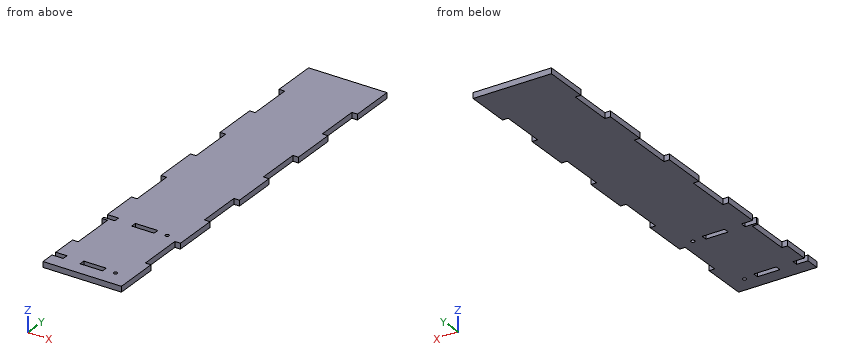
```python
from build123d import *

# Parameters (mm, degrees)
SKETCH2_W           = 6.35
SKETCH2_H           = 88.9
BOSS_EXTRUDE1_DEPTH = 457.2
SKETCH4_W           = 6.35
SKETCH4_H           = 50.8
CUT_EXTRUDE1_DEPTH  = 460.399570091
SKETCH5_W           = 12.7
SKETCH5_H           = 6.35
CUT_EXTRUDE2_DEPTH  = 460.399570091
SKETCH6_R           = 2.0955
CUT_EXTRUDE3_DEPTH  = 460.399570091
SKETCH7_W           = 12.7
SKETCH7_H           = 6.35
CUT_EXTRUDE4_DEPTH  = 10
SKETCH8_W           = 12.7
SKETCH8_H           = 6.35
CUT_EXTRUDE5_DEPTH  = 460.399570091


with BuildPart() as part:
    # Sketch2 → Boss-Extrude1 (new body)
    with BuildSketch(Plane.ZX):
        with Locations((41.275, 0)):
            Rectangle(SKETCH2_W, SKETCH2_H)
    extrude(amount=BOSS_EXTRUDE1_DEPTH)

    # Sketch4 → Cut-Extrude1 (cut, through all)
    with BuildSketch(Plane.XY.offset(44.45)):
        with Locations((41.275, 381)):
            Rectangle(SKETCH4_W, SKETCH4_H)
        with Locations((41.275, 279.4)):
            Rectangle(SKETCH4_W, SKETCH4_H)
        with Locations((41.275, 177.8)):
            Rectangle(SKETCH4_W, SKETCH4_H)
        with Locations((41.275, 76.2)):
            Rectangle(SKETCH4_W, SKETCH4_H)
    cut_extrude1 = extrude(amount=-CUT_EXTRUDE1_DEPTH, mode=Mode.SUBTRACT)

    # Mirror1: Cut-Extrude1 across plane
    add(cut_extrude1.mirror(Plane(origin=(0, 0, 0), x_dir=(0, 0, 1), z_dir=(1, 0, 0))), mode=Mode.SUBTRACT)

    # Sketch5 → Cut-Extrude2 (cut, through all)
    with BuildSketch(Plane(origin=(0, 0, 38.1), x_dir=(-1, 0, 0), z_dir=(0, 0, -1))):
        with Locations((6.35, 18.7625)):
            Rectangle(SKETCH5_W, SKETCH5_H)
        with Locations((-6.35, 18.7625)):
            Rectangle(SKETCH5_W, SKETCH5_H)
        with Locations((6.35, 107.6625)):
            Rectangle(SKETCH5_W, SKETCH5_H)
        with Locations((-6.35, 107.6625)):
            Rectangle(SKETCH5_W, SKETCH5_H)
    extrude(amount=-CUT_EXTRUDE2_DEPTH, mode=Mode.SUBTRACT)

    # Sketch6 → Cut-Extrude3 (cut, through all)
    with BuildSketch(Plane.XY.offset(44.45)):
        with Locations((25.4, 107.6625)):
            Circle(SKETCH6_R)
        with Locations((25.4, 18.7625)):
            Circle(SKETCH6_R)
    extrude(amount=-CUT_EXTRUDE3_DEPTH, mode=Mode.SUBTRACT)

    # Sketch7 → Cut-Extrude4 (cut)
    with BuildSketch(Plane(origin=(0, 0, 38.1), x_dir=(-1, 0, 0), z_dir=(0, 0, -1))):
        with Locations((38.1, 107.6625)):
            Rectangle(SKETCH7_W, SKETCH7_H)
    extrude(amount=-CUT_EXTRUDE4_DEPTH, mode=Mode.SUBTRACT)

    # Sketch8 → Cut-Extrude5 (cut, through all)
    with BuildSketch(Plane(origin=(0, 0, 38.1), x_dir=(-1, 0, 0), z_dir=(0, 0, -1))):
        with Locations((38.1, 18.7625)):
            Rectangle(SKETCH8_W, SKETCH8_H)
    extrude(amount=-CUT_EXTRUDE5_DEPTH, mode=Mode.SUBTRACT)


solid = part.part
```
Build history of the part. All positions in model axes, mm. Coordinates: 2 decimals unless noted, no trailing zeros. Order: outer loops, then holes, each group sorted by start corner. A loop starts at its lowest first (then second) coordinate and runs counter-clockwise, first axis right, second up. Notation, with made-up numbers: (-1, 3.5) -> (49, 3.5) arc R20 cw to (49, 25.5) -> close; hole circle Ø9 at (42, 53). An arc over 180 degrees is marked (long way). Answer in a Markdown table with one row per item. Add a question column.
Q1. Drop flat-ended pins along their axis: pin 1 (3 mm diameter, centred on x = -40.5, z = 39.5, fed in from -Y); pin 2 (3 mm diameter, centred on y = 108, z = 41.5, fed in from -X). Give the stop position or say it passes through.
Q2. Band-saw the part on A-A, the plane y = 393. List the corners of the cut face in (x, z), then the cut area to 3 significant figures.
Q3. Wall check: line 1 along Y through (x, z) = (4, 40); line 2 along Y through (x, z) = (25.4, 39.5); line 3 along Y through (x, z) = (39, 42.5). Give the ranges that are in metal, low to high. Write a range as [from, to].
Q4. Band-saw the part on B-B, the plane z = 40.75. Give the number of separate pieces and of enclosed holes in the cut face, then the cut area to 3 significant figures.
Answers follow:
| question | item | result |
|---|---|---|
| 1 | pin 1 | y = 0 |
| 1 | pin 2 | x = -31.75 |
| 2 | outline | (-38.1, 38.1) -> (38.1, 38.1) -> (38.1, 44.45) -> (-38.1, 44.45) -> close |
| 2 | area | 484 mm^2 |
| 3 | line 1 | [0, 15.59], [21.94, 104.49], [110.84, 457.2] |
| 3 | line 2 | [0, 16.67], [20.86, 105.57], [109.76, 457.2] |
| 3 | line 3 | [0, 50.8], [101.6, 152.4], [203.2, 254], [304.8, 355.6], [406.4, 457.2] |
| 4 | separate pieces | 1 |
| 4 | enclosed holes | 4 |
| 4 | area | 37,600 mm^2 |
